Input: part model. Units: mm. Frame: model coordinates. Give positions to 0.01 mm unless a question says otherwise; leave off trailing zeros. Write each loop counter-clockwise with the first axis right and the second up, starting at its lowest first coordinate (ties: lowest second). Pieces come first, ordered by that corner, then holes.
```python
from build123d import *

# Parameters (mm, degrees)
F0_R     = 4
F1_DEPTH = 10


with BuildPart() as f1:
    # F0 (on Front) → F1 (new body)
    with BuildSketch(Plane.XZ):
        Polygon((0, 300), (0, 0), (80, 0), (80, 130), (60, 190), (60, 300), align=None)
        with Locations((30, 230)):
            Circle(F0_R, mode=Mode.SUBTRACT)
        with Locations((30, 255)):
            Circle(F0_R, mode=Mode.SUBTRACT)
        with Locations((30, 280)):
            Circle(F0_R, mode=Mode.SUBTRACT)
    extrude(amount=-F1_DEPTH)


solid = f1.part
```
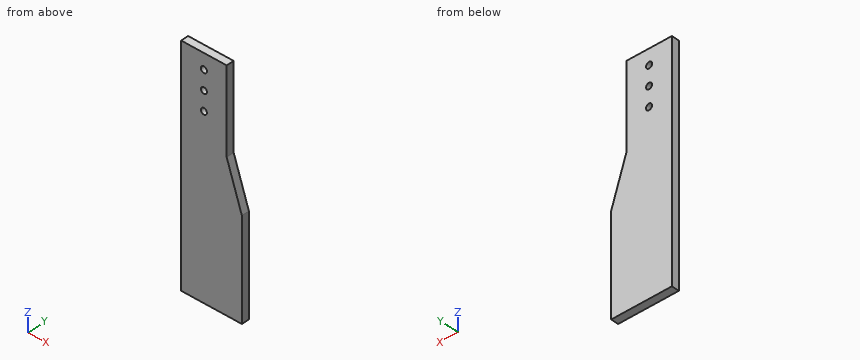
Q1. Material intervals for line 1 along Z through (x, y) = (30, 3); line 2 along X through (y, z) = (3.75, 280); line 3 along Z through (x, y) = (27, 7.25), sorted ascending.
Q2. Section C-C, the plane y = 7. Return the cut outline in (x, z), then the cut area to 3 significant figures.
Q3. Section A-A, the plane x = 30. Return the cut outline in (y, z), then the cut area to 3 significant figures.
Q4. Section D-D, the plane x = 66.5. Return the cut outline in (y, z).
Q5. Section B-B, the plane z = 280. Return the cut outline in (x, y).
Q6. Pin query (flat end, axial travel): pin 1 (3 mm diameter, centred on y = 7, z = 224, fed in from +X); pin 2 (6.5 mm diameter, centred on x = 30, z = 230, fed in from +Y). Return the tip coordinate at first contact, or that it passes through.
Solutions:
1. line 1: z = 0 to 226, 234 to 251, 259 to 276, 284 to 300
1. line 2: x = 0 to 26, 34 to 60
1. line 3: z = 0 to 227.35, 232.65 to 252.35, 257.65 to 277.35, 282.65 to 300
2. outline: (0, 0) - (80, 0) - (80, 130) - (60, 190) - (60, 300) - (0, 300) - close; hole circle Ø8 at (30, 230); hole circle Ø8 at (30, 255); hole circle Ø8 at (30, 280)
2. area: 21,000 mm2
3. outline: (0, 0) - (10, 0) - (10, 226) - (0, 226) - close; (0, 234) - (10, 234) - (10, 251) - (0, 251) - close; (0, 259) - (10, 259) - (10, 276) - (0, 276) - close; (0, 284) - (10, 284) - (10, 300) - (0, 300) - close
3. area: 2,760 mm2
4. outline: (0, 0) - (10, 0) - (10, 170.5) - (0, 170.5) - close
5. outline: (0, 0) - (26, 0) - (26, 10) - (0, 10) - close; (34, 0) - (60, 0) - (60, 10) - (34, 10) - close
6. pin 1: stops at x = 60
6. pin 2: passes through
